Check sheet for the drawn part. Datum: minimum x, y, z corner. Units: mm. A direction names the side the tool comes from. Coordinates: 2 decimals unless noted, no trailing zeros. Write each loop counter-clockwise with the first axis right and the second up, starting at its lowest first coordinate (ties: lowest second). Pieces come first, ordered by that corner, then holes. Notation, with made-up numbers: (60.25, 65.25) - (81.25, 65.25) arc R24 cw to (81.25, 77.25) - close; hole circle Ø9 at (24, 72.25). An arc over 180 degrees is marked (long way). Answer as CSV lines item,"result". Start each with the question number.
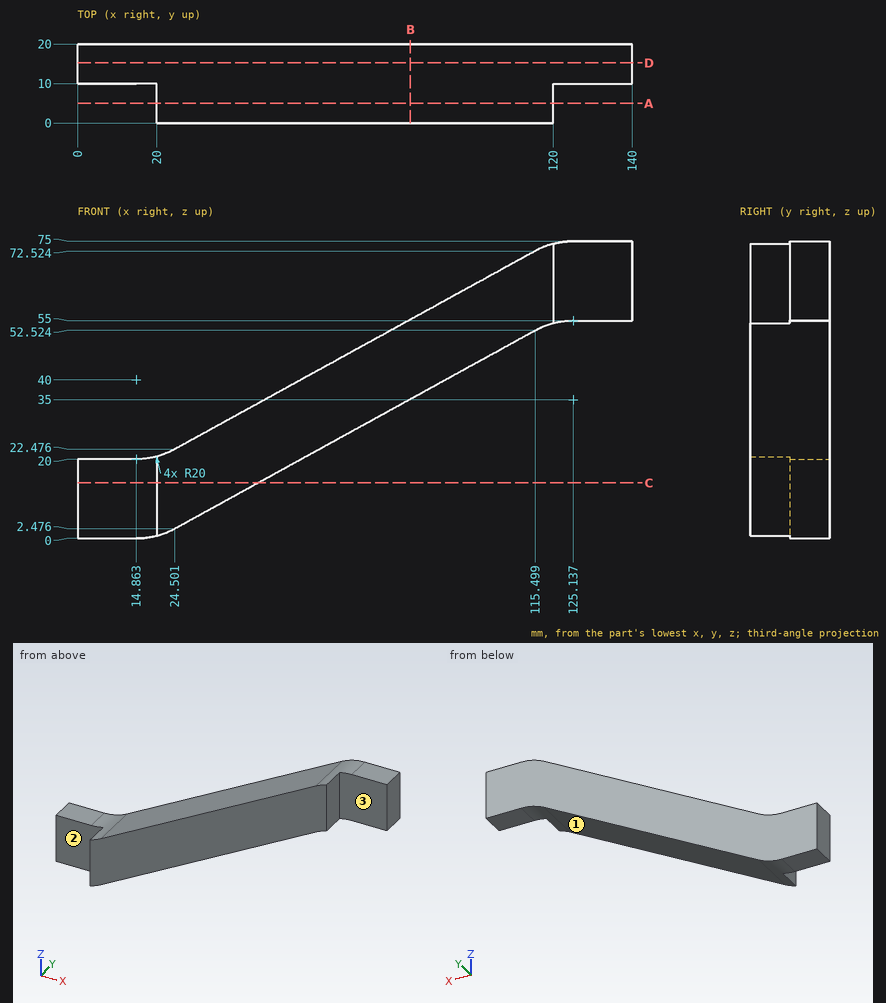
(1) Cross-section at D-D on y = 15.25. Record the boundary of the cut face in (x, z), plus the area to 3 significant figures.
(2) Cross-section at C-C on z = 14. Record the boundary of the cut face in (x, y) (1 decimal), plus the area to 3 significant figures.
(3) Cross-section at A-A on y = 5. Record the boundary of the cut face in (x, z).
(4) Tool access check on the marked faces 1, 2 and 3. Record the directions out of +Z, -Z, +X, -X, +Y, -Y that give a thin tool (end or side, any length) a straight path to the whole face; none if there is none.
(5) Cross-section at B-B on x = 84. Record the boundary of the cut face in (y, z).
(6) Material ranges on probe 1 along Y at (x, z) = (120.5, 65); probe 2 along X at (y, z) = (16.25, 43); probe 3 along X at (y, z) = (12.75, 22), recorded low to high. Write a range as from..to.
(7) Go/stop test with flat-tipped pins: P1, Ø6, axis at x = 81.5, y = 7, coming from the -Z side (1 decimal); P2, Ø8, axis at x = 133, y = 13, coming from the -Z side; P3, Ø11, axis at x = 5, y = 15, coming from the +Z side. Record where each tip stops, or that it passes through.
Checked values:
1,outline,"(0, 0) - (14.86, 0) arc R20 ccw to (24.5, 2.48) - (115.5, 52.52) arc R20 cw to (125.14, 55) - (140, 55) - (140, 75) - (125.14, 75) arc R20 ccw to (115.5, 72.52) - (24.5, 22.48) arc R20 cw to (14.86, 20) - (0, 20) - close"
1,area,"2,800 mm^2"
2,outline,"(0, 10) - (20, 10) - (20, 0) - (45.5, 0) - (45.5, 20) - (0, 20) - close"
2,area,"709 mm^2"
3,outline,"(20, 0.67) arc R20 ccw to (24.5, 2.48) - (115.5, 52.52) arc R20 cw to (120, 54.33) - (120, 74.33) arc R20 ccw to (115.5, 72.52) - (24.5, 22.48) arc R20 cw to (20, 20.67) - close"
4,face 1,"-Z, +X, +Y, -Y"
4,face 2,"+Z, -Z, -X, -Y"
4,face 3,"+Z, -Z, +X, -Y"
5,outline,"(0, 35.2) - (20, 35.2) - (20, 55.2) - (0, 55.2) - close"
6,probe 1,"10..20"
6,probe 2,"61.82..98.18"
6,probe 3,"23.58..60"
7,P1,"z = 32.2"
7,P2,"z = 55"
7,P3,"z = 20"
